```python
from build123d import *

# Parameters (mm, degrees)
F0_W     = 34.200002
F0_H     = 34.200002
F0_W_2   = 32
F0_H_2   = 32
F1_DEPTH = 27.5
F2_R     = 5


with BuildPart() as f1:
    # F0 (on Top) → F1 (new body)
    with BuildSketch(Plane.XY):
        with Locations((-1, 1)):
            Rectangle(F0_W, F0_H)
        with Locations((-1, 1)):
            Rectangle(F0_W_2, F0_H_2, mode=Mode.SUBTRACT)
    extrude(amount=F1_DEPTH)

    # F2
    f2_edges = [f1.edges().sort_by_distance(p)[0] for p in [
        (16.100001, -16.100001, 13.75),
        (16.100001, 18.100001, 13.75),
        (-18.100001, -16.100001, 13.75),
        (-17, 17, 13.75),
        (-17, -15, 13.75),
        (15, -15, 13.75),
        (15, 17, 13.75),
        (-18.100001, 18.100001, 13.75),
    ]]
    fillet(f2_edges, radius=F2_R)


solid = f1.part
```
CAD build for the part. Positions are in the model's coordinates, mm. A direction names the side the tool comes from. Round coordinates to 2 decimals unless told otherwise and drop trailing zeros. Order: outer loops, then holes, each group sorted by start corner. A loop starts at its lowest first (then second) coordinate and runs counter-clockwise, first axis right, second up. Notation, with made-up numbers: (-8, -34.5) - (36, -34.5) arc R18 ccw to (36, -14.5) - close; hole circle Ø6 at (69.5, -18.75). An arc over 180 degrees is marked (long way). Use CSV: the item, a comma, the result in double quotes. Start each with the question number.
1) Two-plate mould, pull along X, no slides. Class faces 3 (the flat face through (-18.1, 1, 14)), 4 (the flat face through (-1, -15, 14)), 5 (the cylindrical face through (-15, -14, 14)), 6 (the flat face through (-2.3, -15.4, 27.5)): pulls with the +X half, pulls with the -X half, needs draft (parallel to the pull), parting line crosses it, or undercut.
2) Saw through at B-B (x = -5.5). List the corners of the cut face in (y, z).
3) Wall check: L1, parallel to Y at x = -2, z = 22; L2, parallel to X at y = 11, z = 24.5; L3, parallel to X at y = -12, z = 5.5. Give the ranges that are in metal, low to high. Write a range as [from, to].
4) Saw through at A-A (y = -4). List the corners of the cut face in (x, z).
5) Saw through at C-C (z = 13.75). List the corners of the cut face in (x, y), and give its area (3 significant figures).
6) Tool access for faces 1 (the flat face through (-17, 1, 14)), 2 (the cylindrical face through (14.6, -14.67, 13.94)): list every direction of +Z, -Z, +X, -X, +Y, -Y with a clear straight run to the whole face (end or side of a thin tool).
Values follow:
1,face 3,"pulls with the -X half"
1,face 4,"undercut"
1,face 5,"undercut"
1,face 6,"needs draft"
2,outline,"(-16.1, 0) - (-15, 0) - (-15, 27.5) - (-16.1, 27.5) - close; (17, 0) - (18.1, 0) - (18.1, 27.5) - (17, 27.5) - close"
3,L1,"y = [-16.1, -15], [17, 18.1]"
3,L2,"x = [-18.1, -17], [15, 16.1]"
3,L3,"x = [-18.02, -16.58], [14.58, 16.02]"
4,outline,"(-18.1, 0) - (-17, 0) - (-17, 27.5) - (-18.1, 27.5) - close; (15, 0) - (16.1, 0) - (16.1, 27.5) - (15, 27.5) - close"
5,outline,"(-18.1, -11.1) arc R5 ccw to (-13.1, -16.1) - (11.1, -16.1) arc R5 ccw to (16.1, -11.1) - (16.1, 13.1) arc R5 ccw to (11.1, 18.1) - (-13.1, 18.1) arc R5 ccw to (-18.1, 13.1) - close; hole (-17, -10) arc R5 ccw to (-12, -15) - (10, -15) arc R5 ccw to (15, -10) - (15, 12) arc R5 ccw to (10, 17) - (-12, 17) arc R5 ccw to (-17, 12) - close"
5,area,"146 mm2"
6,face 1,"+Z, -Z"
6,face 2,"+Z, -Z, +X, -Y"
